Geometry check sheet. Reference: the model listing, model coordinates, mm. Give positions to 0.01 mm unless a question says otherwise; leave off trailing zeros. Loops run counter-clockwise (first coordinate to the right, second up) from the corner with the lowest first, then second, coordinate; pieces in that order, holes last. Notation, with made-up numbers: (-29, 4) - (-14, 4) arc R17 cw to (-14, 33) - close; hole circle Ø2 at (88.25, -22.5). An arc over 180 degrees is marked (long way). Write item = value, one per line. Start each with the question number.
Autodesk Inventor part; units mm, degrees
ref_plane "作業平面1" through (0, 0, 0) normal (0, 0, 1) x (1, 0, 0)
ref_plane "YZ Plane" through (0, 0, 0) normal (1, 0, 0) x (0, 1, 0)
ref_plane "XZ Plane" through (0, 0, 0) normal (0, 1, 0) x (-1, 0, 0)
ref_plane "作業平面1" through (0, 0, 0) normal (0, 0, 1) x (1, 0, 0)
sketch "スケッチ1" plane through (0, 0, 0) normal (0, 0, 1) x (1, 0, 0)
  circle A0 centre (-14.624772, 63.539385) radius 64
  arc A1 (-81.893775, 52.547912) -> (-80.479561, 53.962126) centre (-81.186668, 53.255019) ccw
  line L0 (-81.893775, 52.547912) -> (-83.065348, 52.547912)
  arc A2 (-84.479561, 53.962126) -> (-83.065348, 52.547912) centre (-83.772455, 53.255019) ccw
  line L1 (-84.479561, 53.962126) -> (-84.479561, 73.133699)
  arc A3 (-83.065348, 74.547912) -> (-84.479561, 73.133699) centre (-83.772455, 73.840806) ccw
  line L2 (-83.065348, 74.547912) -> (-81.893775, 74.547912)
  arc A4 (-80.479561, 73.133699) -> (-81.893775, 74.547912) centre (-81.186668, 73.840806) ccw
  line L3 (-80.479561, 73.133699) -> (-80.479561, 53.962126)
  arc A5 (-3.479561, 132.133699) -> (-4.893775, 133.547912) centre (-4.186668, 132.840806) ccw
  line L4 (-3.479561, 132.133699) -> (-3.479561, 130.962126)
  arc A6 (-4.893775, 129.547912) -> (-3.479561, 130.962126) centre (-4.186668, 130.255019) ccw
  line L5 (-4.893775, 129.547912) -> (-24.065348, 129.547912)
  arc A7 (-25.479561, 130.962126) -> (-24.065348, 129.547912) centre (-24.772455, 130.255019) ccw
  line L6 (-25.479561, 130.962126) -> (-25.479561, 132.133699)
  arc A8 (-24.065348, 133.547912) -> (-25.479561, 132.133699) centre (-24.772455, 132.840806) ccw
  line L7 (-24.065348, 133.547912) -> (-4.893775, 133.547912)
  arc A9 (54.106225, 52.547912) -> (55.520439, 53.962126) centre (54.813332, 53.255019) ccw
  line L8 (54.106225, 52.547912) -> (52.934652, 52.547912)
  arc A10 (51.520439, 53.962126) -> (52.934652, 52.547912) centre (52.227545, 53.255019) ccw
  line L9 (51.520439, 53.962126) -> (51.520439, 73.133699)
  arc A11 (52.934652, 74.547912) -> (51.520439, 73.133699) centre (52.227545, 73.840806) ccw
  line L10 (52.934652, 74.547912) -> (54.106225, 74.547912)
  arc A12 (55.520439, 73.133699) -> (54.106225, 74.547912) centre (54.813332, 73.840806) ccw
  line L11 (55.520439, 73.133699) -> (55.520439, 53.962126)
  arc A13 (-25.479561, -5.037874) -> (-24.065348, -6.452088) centre (-24.772455, -5.744981) ccw
  line L12 (-25.479561, -5.037874) -> (-25.479561, -3.866301)
  arc A14 (-24.065348, -2.452088) -> (-25.479561, -3.866301) centre (-24.772455, -3.159194) ccw
  line L13 (-24.065348, -2.452088) -> (-4.893775, -2.452088)
  arc A15 (-3.479561, -3.866301) -> (-4.893775, -2.452088) centre (-4.186668, -3.159194) ccw
  line L14 (-3.479561, -3.866301) -> (-3.479561, -5.037874)
  arc A16 (-4.893775, -6.452088) -> (-3.479561, -5.037874) centre (-4.186668, -5.744981) ccw
  line L15 (-4.893775, -6.452088) -> (-24.065348, -6.452088)
  arc A17 (-90.380937, 104.093949) -> (-92.776199, 103.718007) centre (-91.441598, 103.033289) ccw
  arc A18 (-92.776199, 103.718007) -> (-98.248191, 90.50745) centre (-14.479561, 63.547912) ccw
  arc A19 (-98.248191, 90.50745) -> (-96.820317, 88.547912) centre (-96.820317, 90.047912) ccw
  line L16 (-96.820317, 88.547912) -> (-88.479561, 88.547912)
  arc A20 (-86.479561, 86.547912) -> (-88.479561, 88.547912) centre (-88.479561, 86.547912) ccw
  line L17 (-86.479561, 86.547912) -> (-86.479561, 40.547912)
  arc A21 (-88.479561, 38.547912) -> (-86.479561, 40.547912) centre (-88.479561, 40.547912) ccw
  line L18 (-88.479561, 38.547912) -> (-96.820317, 38.547912)
  arc A22 (-96.820317, 38.547912) -> (-98.248191, 36.588375) centre (-96.820317, 37.047912) ccw
  arc A23 (-98.248191, 36.588375) -> (-41.439099, -20.220717) centre (-14.479561, 63.547912) ccw
  arc A24 (-41.439099, -20.220717) -> (-39.479561, -18.792843) centre (-40.979561, -18.792843) ccw
  line L19 (-39.479561, -18.792843) -> (-39.479561, -10.452088)
  arc A25 (-37.479561, -8.452088) -> (-39.479561, -10.452088) centre (-37.479561, -10.452088) ccw
  line L20 (-37.479561, -8.452088) -> (8.520439, -8.452088)
  arc A26 (10.520439, -10.452088) -> (8.520439, -8.452088) centre (8.520439, -10.452088) ccw
  line L21 (10.520439, -10.452088) -> (10.520439, -18.792843)
  arc A27 (10.520439, -18.792843) -> (12.479976, -20.220717) centre (12.020439, -18.792843) ccw
  arc A28 (12.479976, -20.220717) -> (25.690533, -14.748726) centre (-14.479561, 63.547912) ccw
  arc A29 (25.690533, -14.748726) -> (26.066476, -12.353464) centre (25.005815, -13.414124) ccw
  line L22 (26.066476, -12.353464) -> (20.079693, -6.366681)
  arc A30 (20.079693, -2.124041) -> (20.079693, -6.366681) centre (22.201014, -4.245361) ccw
  line L23 (20.079693, -2.124041) -> (22.554567, 0.350833)
  arc A31 (55.435032, 28.988658) -> (51.192392, 28.988658) centre (53.313712, 26.867337) ccw
  line L24 (55.435032, 28.988658) -> (61.421815, 23.001875)
  arc A32 (61.421815, 23.001875) -> (63.817077, 23.377818) centre (62.482475, 24.062536) ccw
  arc A33 (63.817077, 23.377818) -> (69.289068, 36.588375) centre (-14.479561, 63.547912) ccw
  arc A34 (69.289068, 36.588375) -> (67.861194, 38.547912) centre (67.861194, 37.047912) ccw
  line L25 (67.861194, 38.547912) -> (59.520439, 38.547912)
  arc A35 (57.520439, 40.547912) -> (59.520439, 38.547912) centre (59.520439, 40.547912) ccw
  line L26 (57.520439, 40.547912) -> (57.520439, 86.547912)
  arc A36 (59.520439, 88.547912) -> (57.520439, 86.547912) centre (59.520439, 86.547912) ccw
  line L27 (59.520439, 88.547912) -> (67.861194, 88.547912)
  arc A37 (67.861194, 88.547912) -> (69.289068, 90.50745) centre (67.861194, 90.047912) ccw
  arc A38 (69.289068, 90.50745) -> (12.479976, 147.316542) centre (-14.479561, 63.547912) ccw
  arc A39 (12.479976, 147.316542) -> (10.520439, 145.888668) centre (12.020439, 145.888668) ccw
  line L28 (10.520439, 145.888668) -> (10.520439, 137.547912)
  arc A40 (8.520439, 135.547912) -> (10.520439, 137.547912) centre (8.520439, 137.547912) ccw
  line L29 (8.520439, 135.547912) -> (-37.479561, 135.547912)
  arc A41 (-39.479561, 137.547912) -> (-37.479561, 135.547912) centre (-37.479561, 137.547912) ccw
  line L30 (-39.479561, 137.547912) -> (-39.479561, 145.888668)
  arc A42 (-39.479561, 145.888668) -> (-41.439099, 147.316542) centre (-40.979561, 145.888668) ccw
  arc A43 (-41.439099, 147.316542) -> (-54.649656, 141.84455) centre (-14.479561, 63.547912) ccw
  arc A44 (-54.649656, 141.84455) -> (-55.025598, 139.449288) centre (-53.964938, 140.509949) ccw
  line L31 (-55.025598, 139.449288) -> (-49.038816, 133.462506)
  arc A45 (-49.038816, 129.219865) -> (-49.038816, 133.462506) centre (-51.160136, 131.341186) ccw
  line L32 (-54.342117, 123.916565) -> (-74.848214, 103.410468)
  arc A46 (-84.394155, 98.107167) -> (-80.151514, 98.107167) centre (-82.272835, 100.228487) ccw
  line L33 (-84.394155, 98.107167) -> (-90.380937, 104.093949)
  arc A47 (-32.657783, 124.912008) -> (-31.62228, 126.687656) centre (-33.083835, 126.350229) ccw
  line L34 (-31.62228, 126.687656) -> (-31.649781, 126.806774)
  arc A48 (-26.77793, 127.931529) -> (-31.649781, 126.806774) centre (-29.213855, 127.369152) ccw
  line L35 (-26.77793, 127.931529) -> (-26.75043, 127.812411)
  arc A49 (-26.75043, 127.812411) -> (-25.041333, 126.670404) centre (-25.288875, 128.149838) ccw
  arc A50 (48.642931, 52.986141) -> (-25.041333, 126.670404) centre (-14.479561, 63.547912) ccw
  arc A51 (48.642931, 52.986141) -> (49.784937, 51.277044) centre (50.122364, 52.738599) ccw
  line L36 (49.784937, 51.277044) -> (49.904056, 51.249544)
  arc A52 (48.7793, 46.377693) -> (49.904056, 51.249544) centre (49.341678, 48.813618) ccw
  line L37 (48.7793, 46.377693) -> (48.660182, 46.405194)
  arc A53 (48.660182, 46.405194) -> (46.884535, 45.369691) centre (48.322756, 44.943639) ccw
  arc A54 (3.69866, 2.183817) -> (46.884535, 45.369691) centre (-14.479561, 63.547912) ccw
  arc A55 (3.69866, 2.183817) -> (2.663157, 0.408169) centre (4.124712, 0.745596) ccw
  line L38 (2.663157, 0.408169) -> (2.690658, 0.289051)
  arc A56 (-2.181192, -0.835704) -> (2.690658, 0.289051) centre (0.254733, -0.273327) ccw
  line L39 (-2.181192, -0.835704) -> (-2.208693, -0.716586)
  arc A57 (-2.208693, -0.716586) -> (-3.91779, 0.425421) centre (-3.670248, -1.054013) ccw
  arc A58 (-77.602053, 74.109684) -> (-3.91779, 0.425421) centre (-14.479561, 63.547912) ccw
  arc A59 (-77.602053, 74.109684) -> (-78.74406, 75.818781) centre (-79.081487, 74.357226) ccw
  line L40 (-78.74406, 75.818781) -> (-78.863178, 75.846281)
  arc A60 (-77.738423, 80.718132) -> (-78.863178, 75.846281) centre (-78.300801, 78.282206) ccw
  line L41 (-77.738423, 80.718132) -> (-77.619305, 80.690631)
  arc A61 (-77.619305, 80.690631) -> (-75.843657, 81.726134) centre (-77.281878, 82.152186) ccw
  arc A62 (-32.657783, 124.912008) -> (-75.843657, 81.726134) centre (-14.479561, 63.547912) ccw
  circle A63 centre (65.069166, 92.047912) radius 2.5
  circle A64 centre (-42.979561, -16.000815) radius 2.5
  circle A65 centre (14.020439, 143.09664) radius 2.5
  circle A66 centre (-94.028289, 35.047912) radius 2.5
  circle A67 centre (49.341678, 48.813618) radius 1
  circle A68 centre (0.254733, -0.273327) radius 1
  circle A69 centre (-78.300801, 78.282206) radius 1
  circle A70 centre (-29.213855, 127.369152) radius 1
  circle A71 centre (-14.479561, 63.547912) radius 55
  circle A72 centre (19.135053, 141.074087) radius 2
  circle A73 centre (63.046613, 97.162527) radius 2
  circle A74 centre (2.020439, 127.968406) radius 2
  circle A75 centre (49.940932, 80.047912) radius 2
  line L42 (-74.848214, 103.410468) -> (-72.019786, 100.582041)
  line L43 (-71.31268, 99.874934) -> (-74.141107, 97.046507)
  line L44 (-74.848214, 97.753614) -> (-77.676641, 100.582041)
  line L45 (-49.038816, 129.219865) -> (-51.51369, 126.744992)
  line L46 (-51.51369, 126.744992) -> (-48.685263, 123.916565)
  line L47 (-47.978156, 123.209458) -> (-50.806583, 120.381031)
  line L48 (-51.51369, 121.088137) -> (-54.342117, 123.916565)
  arc A76 (-47.978156, 123.209458) -> (-48.685263, 123.916565) centre (-48.331709, 123.563011) ccw
  arc A77 (-51.51369, 121.088137) -> (-50.806583, 120.381031) centre (-51.160136, 120.734584) ccw
  arc A78 (-71.31268, 99.874934) -> (-72.019786, 100.582041) centre (-71.666233, 100.228487) ccw
  arc A79 (-74.848214, 97.753614) -> (-74.141107, 97.046507) centre (-74.49466, 97.40006) ccw
  line L49 (-77.676641, 100.582041) -> (-80.151514, 98.107167)
  line L50 (22.554567, 0.350833) -> (19.72614, 3.17926)
  arc A80 (19.019033, 3.886367) -> (19.72614, 3.17926) centre (19.372587, 3.532814) ccw
  line L51 (19.019033, 3.886367) -> (21.84746, 6.714794)
  arc A81 (22.554567, 6.007687) -> (21.84746, 6.714794) centre (22.201014, 6.361241) ccw
  line L52 (22.554567, 6.007687) -> (25.382994, 3.17926)
  line L53 (25.382994, 3.17926) -> (45.889091, 23.685357)
  line L54 (45.889091, 23.685357) -> (43.060664, 26.513784)
  arc A82 (42.353557, 27.220891) -> (43.060664, 26.513784) centre (42.70711, 26.867337) ccw
  line L55 (42.353557, 27.220891) -> (45.181984, 30.049318)
  arc A83 (45.889091, 29.342211) -> (45.181984, 30.049318) centre (45.535537, 29.695765) ccw
  line L56 (45.889091, 29.342211) -> (48.717518, 26.513784)
  line L57 (48.717518, 26.513784) -> (51.192392, 28.988658)
  point P0 (0, 0)
  dimension "d0" = 2
  dimension "d3" = 110
sketch "スケッチ1 outline for 押し出し1" plane through (0, 0, 0) normal (0, 0, 1) x (1, 0, 0)
  line L0 (-78.863178, 75.846281) -> (-78.74406, 75.818781)
  arc A0 (-77.738423, 80.718132) -> (-78.863178, 75.846281) centre (-78.300801, 78.282206) ccw
  arc A1 (-78.74406, 75.818781) -> (-77.602053, 74.109684) centre (-79.081487, 74.357226) cw
  line L1 (-77.619305, 80.690631) -> (-77.738423, 80.718132)
  arc A2 (-77.602053, 74.109684) -> (-3.91779, 0.425421) centre (-14.479561, 63.547912) ccw
  arc A3 (-75.843657, 81.726134) -> (-77.619305, 80.690631) centre (-77.281878, 82.152186) cw
  arc A4 (-3.91779, 0.425421) -> (-2.208693, -0.716586) centre (-3.670248, -1.054013) cw
  arc A5 (-32.657783, 124.912008) -> (-75.843657, 81.726134) centre (-14.479561, 63.547912) ccw
  line L2 (-2.208693, -0.716586) -> (-2.181192, -0.835704)
  arc A6 (-31.62228, 126.687656) -> (-32.657783, 124.912008) centre (-33.083835, 126.350229) cw
  arc A7 (-2.181192, -0.835704) -> (2.690658, 0.289051) centre (0.254733, -0.273327) ccw
  line L3 (-31.649781, 126.806774) -> (-31.62228, 126.687656)
  line L4 (2.690658, 0.289051) -> (2.663157, 0.408169)
  arc A8 (-26.77793, 127.931529) -> (-31.649781, 126.806774) centre (-29.213855, 127.369152) ccw
  arc A9 (2.663157, 0.408169) -> (3.69866, 2.183817) centre (4.124712, 0.745596) cw
  line L5 (-26.75043, 127.812411) -> (-26.77793, 127.931529)
  arc A10 (3.69866, 2.183817) -> (46.884535, 45.369691) centre (-14.479561, 63.547912) ccw
  arc A11 (-25.041333, 126.670404) -> (-26.75043, 127.812411) centre (-25.288875, 128.149838) cw
  arc A12 (46.884535, 45.369691) -> (48.660182, 46.405194) centre (48.322756, 44.943639) cw
  arc A13 (48.642931, 52.986141) -> (-25.041333, 126.670404) centre (-14.479561, 63.547912) ccw
  line L6 (48.660182, 46.405194) -> (48.7793, 46.377693)
  arc A14 (49.784937, 51.277044) -> (48.642931, 52.986141) centre (50.122364, 52.738599) cw
  arc A15 (48.7793, 46.377693) -> (49.904056, 51.249544) centre (49.341678, 48.813618) ccw
  line L7 (49.904056, 51.249544) -> (49.784937, 51.277044)
  circle A16 centre (0.254733, -0.273327) radius 1
  circle A17 centre (-14.479561, 63.547912) radius 55
  circle A18 centre (49.341678, 48.813618) radius 1
  circle A19 centre (-78.300801, 78.282206) radius 1
  circle A20 centre (-29.213855, 127.369152) radius 1
extrude "押し出し1" add sketch "スケッチ1 outline for 押し出し1" along normal blind 1.2
properties part number "LineSensor"
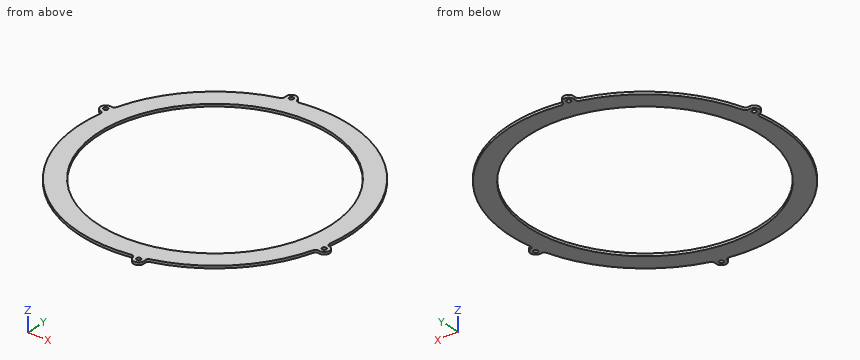
1) Cross-section at B-B on z = 0.85. Give the number of separate pieces and of enclosed holes in the cut face, and give its area (3 significant figures).
2) Cross-section at A-A on x = 13.5. Enter the section's corners in (y, z).
3) Cross-section at C-C on y = 12. Enter the section's corners in (x, z), and give its area (3 significant figures).
4) Material ranges on line 1 along Y through (x, z) = (-13, 0.65); line 2 along Y through (x, z) = (-29, 0.35); line 3 along Y through (x, z) = (28.5, 0.95), recorded low to high.
Checked values:
q1.separate_pieces = 1
q1.enclosed_holes = 5
q1.area = 3,430 mm²
q2.outline = (5.99, 0) - (16.2, 0) - (16.2, 1.2) - (5.99, 1.2) - close; (110.9, 0) - (121.11, 0) - (121.11, 1.2) - (110.9, 1.2) - close
q3.outline = (-52.41, 0) - (-33.66, 0) - (-33.66, 1.2) - (-52.41, 1.2) - close; (4.7, 0) - (23.45, 0) - (23.45, 1.2) - (4.7, 1.2) - close
q3.area = 45.0 mm²
q4.line_1 = -0.43 to 8.57, 118.53 to 127.53
q4.line_2 = 1.22 to 10.5, 116.6 to 126.39, 128.35 to 129.86
q4.line_3 = 16.13 to 29.23, 97.87 to 110.97
